The drawing under review shows one solid part. Ordinate dimensions are in mm from its lowest x, y, z. Round coordinates to 2 decimals unless told otherwise and drop trailing zeros. Write each loop counter-clockwise with the first axis right and the second up, starting at its lowest first coordinate (ties: lowest second). Pieces come first, ordered by that corner, then holes.
Item 1: To check wall thickness, follow L1, parallel to Y at x = 17, z = 0.6; L2, parallel to X at y = 26.5, z = 2.45; L3, parallel to X at y = 15, z = 0.1. State the ranges of each line that lie inside material, in increasing order.
Item 2: Add section C-C (x = 93). Give the boundary of the cut face in (y, z).
Item 3: Add section B-B (y = 17). Give the boundary of the cut face in (x, z), plus the area to 3 significant figures.
Item 4: Clearance check with flat-ended pins moving along their axes: pin 1 Ø1 at (x, z) = (68.5, 1) entering from +Y; pin 2 Ø1 at (x, z) = (28, 0.5) entering from -Y. State where each tip first meets the part, or that it passes through.
Item 5: Add section D-D (y = 24). Give the boundary of the cut face in (x, z), plus the area to 3 significant figures.
Item 6: Add section A-A (z = 1.55). Give the boundary of the cut face in (x, y), plus the area to 3 significant figures.
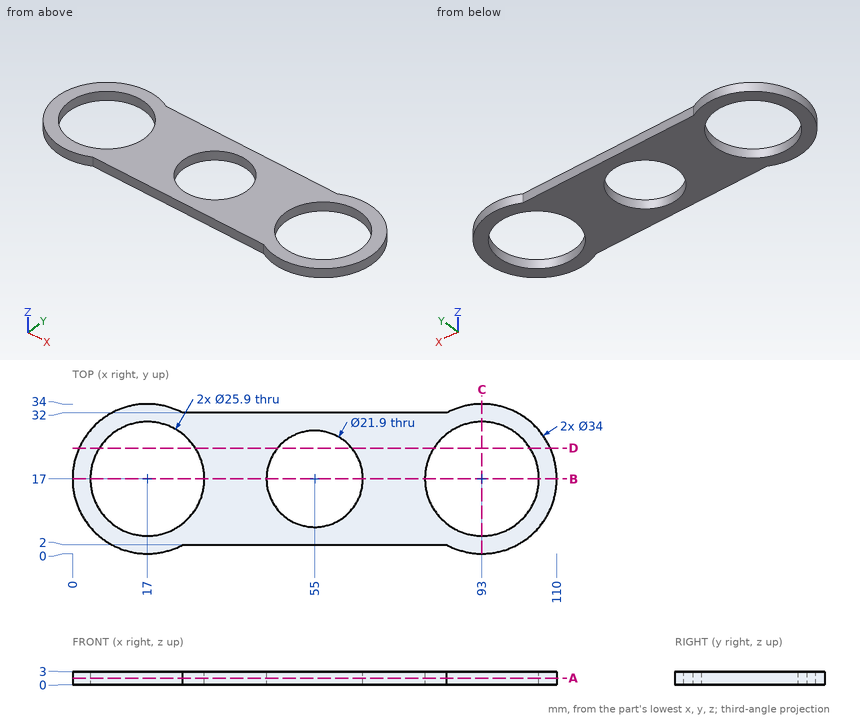
Numbers:
1. L1: y = 0 to 4.05, 29.95 to 34
1. L2: x = 2.9 to 8.2, 25.8 to 49.55, 60.45 to 84.2, 101.8 to 107.1
1. L3: x = 0.12 to 4.21, 29.79 to 44.23, 65.77 to 80.21, 105.79 to 109.88
2. outline: (0, 0) - (4.05, 0) - (4.05, 3) - (0, 3) - close; (29.95, 0) - (34, 0) - (34, 3) - (29.95, 3) - close
3. outline: (0, 0) - (4.05, 0) - (4.05, 3) - (0, 3) - close; (29.95, 0) - (44.05, 0) - (44.05, 3) - (29.95, 3) - close; (65.95, 0) - (80.05, 0) - (80.05, 3) - (65.95, 3) - close; (105.95, 0) - (110, 0) - (110, 3) - (105.95, 3) - close
3. area: 109 mm2
4. pin 1: stops at y = 32
4. pin 2: stops at y = 2
5. outline: (1.51, 0) - (6.1, 0) - (6.1, 3) - (1.51, 3) - close; (27.9, 0) - (46.58, 0) - (46.58, 3) - (27.9, 3) - close; (63.42, 0) - (82.1, 0) - (82.1, 3) - (63.42, 3) - close; (103.9, 0) - (108.49, 0) - (108.49, 3) - (103.9, 3) - close
5. area: 140 mm2
6. outline: (25, 2) - (85, 2) arc R17 ccw (long way) to (85, 32) - (25, 32) arc R17 ccw (long way) to start; hole circle Ø25.9 at (17, 17); hole circle Ø21.9 at (55, 17); hole circle Ø25.9 at (93, 17)
6. area: 1,800 mm2
